Can you work these out from the model? Positions are in its coordinate system, mm. Give positions to 0.01 mm unless a question says otherwise; leave off trailing zeros. Write each loop counter-clockwise with the first axis right and the second up, starting at its lowest first coordinate (ties: lowest second). Pieces come first, ordered by that corner, then holes. Notation, with made-up numbers: (54.25, 4) -> (95.25, 4) arc R11 ccw to (95.25, 11) -> close; hole circle Ø9 at (49, 6). An arc over 180 degrees is marked (long way). One line per item, written item: value.
from build123d import *

# Parameters (mm, degrees)
SKETCH_W               = 190
SKETCH_H               = 132
PAD_DEPTH              = 10
SKETCH001_R            = 2.75
HOLE_DEPTH             = 10.001
LINEARPATTERN_COUNT    = 2
LINEARPATTERN_PITCH    = 60
LINEARPATTERN001_COUNT = 2
LINEARPATTERN001_PITCH = 122
HOLE001_D              = 6.6
HOLE001_CSINK_D        = 12
HOLE001_CSINK_ANGLE    = 90
LINEARPATTERN002_COUNT = 2
LINEARPATTERN002_PITCH = 40
LINEARPATTERN003_COUNT = 2
LINEARPATTERN003_PITCH = 170
LINEARPATTERN004_COUNT = 2
LINEARPATTERN004_PITCH = 130
HOLE002_D              = 6.6
HOLE002_CSINK_D        = 12
HOLE002_CSINK_ANGLE    = 90
LINEARPATTERN005_COUNT = 2
LINEARPATTERN005_PITCH = 40
LINEARPATTERN006_COUNT = 2
LINEARPATTERN006_PITCH = 130
LINEARPATTERN007_COUNT = 2
LINEARPATTERN007_PITCH = 170
HOLE003_D              = 6.6
HOLE003_CSINK_D        = 12
HOLE003_CSINK_ANGLE    = 90
LINEARPATTERN008_COUNT = 2
LINEARPATTERN008_PITCH = 40
LINEARPATTERN009_COUNT = 2
LINEARPATTERN009_PITCH = 130
LINEARPATTERN010_COUNT = 2
LINEARPATTERN010_PITCH = 170
SKETCH005_R            = 2.75
HOLE004_DEPTH          = 10.001
HOLE005_D              = 6.6
HOLE005_CSINK_D        = 12
HOLE005_CSINK_ANGLE    = 90
LINEARPATTERN011_COUNT = 2
LINEARPATTERN011_PITCH = 40
LINEARPATTERN012_COUNT = 2
LINEARPATTERN012_PITCH = 130
LINEARPATTERN013_COUNT = 2
LINEARPATTERN013_PITCH = 170
HOLE006_D              = 5.5
HOLE006_CSINK_D        = 10
HOLE006_CSINK_ANGLE    = 90
LINEARPATTERN014_COUNT = 2
LINEARPATTERN014_PITCH = 40
LINEARPATTERN015_COUNT = 2
LINEARPATTERN015_PITCH = 22
HOLE007_D              = 5.5
HOLE007_CSINK_D        = 10
HOLE007_CSINK_ANGLE    = 90


with BuildPart() as part:
    # Sketch → Pad (new body)
    with BuildSketch(Plane.XY):
        with Locations((95, 66)):
            Rectangle(SKETCH_W, SKETCH_H)
    extrude(amount=PAD_DEPTH)

    # Sketch001 (on Face6 of Pad) → Hole (cut, through all)
    with BuildSketch(Plane.XY.offset(10)):
        with Locations((65, 5)):
            Circle(SKETCH001_R)
    hole = extrude(amount=-HOLE_DEPTH, mode=Mode.SUBTRACT)

    # LinearPattern: Hole ×2
    with Locations(*[(i * LINEARPATTERN_PITCH, 0, 0) for i in range(1, LINEARPATTERN_COUNT)]):
        add(hole, mode=Mode.SUBTRACT)

    # LinearPattern001: Hole ×2
    with Locations(*[(0, i * LINEARPATTERN001_PITCH, 0) for i in range(1, LINEARPATTERN001_COUNT)]):
        add(hole, mode=Mode.SUBTRACT)

    # Hole001 (through all)
    with Locations(Plane.XY.offset(10)):
        with Locations((10, 18)):
            hole001 = CounterSinkHole(HOLE001_D / 2, HOLE001_CSINK_D / 2, counter_sink_angle=HOLE001_CSINK_ANGLE)

    # LinearPattern002: Hole001 ×2
    with Locations(*[(i * LINEARPATTERN002_PITCH, 0, 0) for i in range(1, LINEARPATTERN002_COUNT)]):
        add(hole001, mode=Mode.SUBTRACT)

    # LinearPattern003: Hole001 ×2
    with Locations(*[(i * LINEARPATTERN003_PITCH, 0, 0) for i in range(1, LINEARPATTERN003_COUNT)]):
        add(hole001, mode=Mode.SUBTRACT)

    # LinearPattern004: Hole001 ×2
    with Locations(*[(i * LINEARPATTERN004_PITCH, 0, 0) for i in range(1, LINEARPATTERN004_COUNT)]):
        add(hole001, mode=Mode.SUBTRACT)

    # Hole002 (through all)
    with Locations(Plane.XY.offset(10)):
        with Locations((10, 58)):
            hole002 = CounterSinkHole(HOLE002_D / 2, HOLE002_CSINK_D / 2, counter_sink_angle=HOLE002_CSINK_ANGLE)

    # LinearPattern005: Hole002 ×2
    with Locations(*[(i * LINEARPATTERN005_PITCH, 0, 0) for i in range(1, LINEARPATTERN005_COUNT)]):
        add(hole002, mode=Mode.SUBTRACT)

    # LinearPattern006: Hole002 ×2
    with Locations(*[(i * LINEARPATTERN006_PITCH, 0, 0) for i in range(1, LINEARPATTERN006_COUNT)]):
        add(hole002, mode=Mode.SUBTRACT)

    # LinearPattern007: Hole002 ×2
    with Locations(*[(i * LINEARPATTERN007_PITCH, 0, 0) for i in range(1, LINEARPATTERN007_COUNT)]):
        add(hole002, mode=Mode.SUBTRACT)

    # Hole003 (through all)
    with Locations(Plane.XY.offset(10)):
        with Locations((10, 114)):
            hole003 = CounterSinkHole(HOLE003_D / 2, HOLE003_CSINK_D / 2, counter_sink_angle=HOLE003_CSINK_ANGLE)

    # LinearPattern008: Hole003 ×2
    with Locations(*[(i * LINEARPATTERN008_PITCH, 0, 0) for i in range(1, LINEARPATTERN008_COUNT)]):
        add(hole003, mode=Mode.SUBTRACT)

    # LinearPattern009: Hole003 ×2
    with Locations(*[(i * LINEARPATTERN009_PITCH, 0, 0) for i in range(1, LINEARPATTERN009_COUNT)]):
        add(hole003, mode=Mode.SUBTRACT)

    # LinearPattern010: Hole003 ×2
    with Locations(*[(i * LINEARPATTERN010_PITCH, 0, 0) for i in range(1, LINEARPATTERN010_COUNT)]):
        add(hole003, mode=Mode.SUBTRACT)

    # Sketch005 (on Face5 of LinearPattern010) → Hole004 (cut, through all)
    with BuildSketch(Plane.XY.offset(10)):
        with Locations((125, 127)):
            Circle(SKETCH005_R)
    extrude(amount=-HOLE004_DEPTH, mode=Mode.SUBTRACT)

    # Hole005 (through all)
    with Locations(Plane.XY.offset(10)):
        with Locations((10, 74)):
            hole005 = CounterSinkHole(HOLE005_D / 2, HOLE005_CSINK_D / 2, counter_sink_angle=HOLE005_CSINK_ANGLE)

    # LinearPattern011: Hole005 ×2
    with Locations(*[(i * LINEARPATTERN011_PITCH, 0, 0) for i in range(1, LINEARPATTERN011_COUNT)]):
        add(hole005, mode=Mode.SUBTRACT)

    # LinearPattern012: Hole005 ×2
    with Locations(*[(i * LINEARPATTERN012_PITCH, 0, 0) for i in range(1, LINEARPATTERN012_COUNT)]):
        add(hole005, mode=Mode.SUBTRACT)

    # LinearPattern013: Hole005 ×2
    with Locations(*[(i * LINEARPATTERN013_PITCH, 0, 0) for i in range(1, LINEARPATTERN013_COUNT)]):
        add(hole005, mode=Mode.SUBTRACT)

    # Hole006 (through all)
    with Locations(Plane.XY.offset(10)):
        with Locations((75, 55)):
            hole006 = CounterSinkHole(HOLE006_D / 2, HOLE006_CSINK_D / 2, counter_sink_angle=HOLE006_CSINK_ANGLE)

    # LinearPattern014: Hole006 ×2
    with Locations(*[(i * LINEARPATTERN014_PITCH, 0, 0) for i in range(1, LINEARPATTERN014_COUNT)]):
        add(hole006, mode=Mode.SUBTRACT)

    # LinearPattern015: Hole006 ×2
    with Locations(*[(0, i * LINEARPATTERN015_PITCH, 0) for i in range(1, LINEARPATTERN015_COUNT)]):
        add(hole006, mode=Mode.SUBTRACT)

    # Hole007 (through all)
    with Locations(Plane.XY.offset(10)):
        with Locations((115, 77)):
            CounterSinkHole(HOLE007_D / 2, HOLE007_CSINK_D / 2, counter_sink_angle=HOLE007_CSINK_ANGLE)


solid = part.part
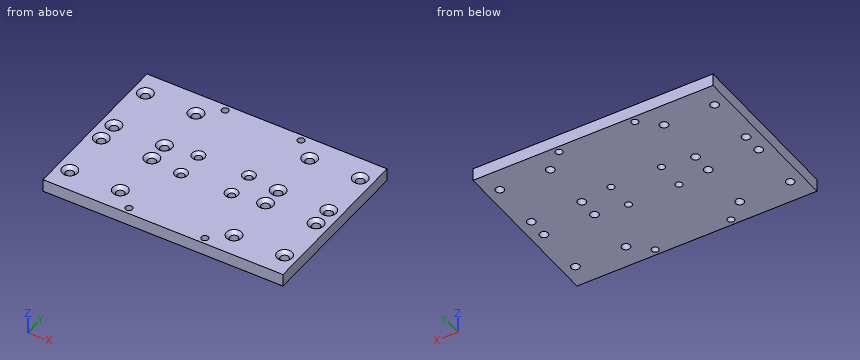
1) Will these pins go through, and if not, where does the flat tip stop? pin 1 (5 mm diameter, centred on x = 94.5, z = 5.5, fed in from -Y); pin 2 (10.5 mm diameter, centred on x = 50, y = 74, fed in from +Z); pin 3 (8.5 mm diameter, centred on x = 180, y = 74, fed in from +Z); pin 4 (7 mm diameter, centred on x = 115, y = 55, fed in from +Z).
Answer list:
pin 1: stops at y = 0
pin 2: stops at z = 9.25
pin 3: stops at z = 8.25
pin 4: stops at z = 8.5
2) If we section it at D-D (z = 4.75): State how many separate pieces and enclosed holes the cut face has, and give its area (3 significant figures).
Answer list:
separate pieces: 1
enclosed holes: 24
area: 24,300 mm^2
3) If we section it at B-B (y = 114): Write out the boundary of the cut face in (x, z).
Answer list:
outline: (0, 0) -> (6.7, 0) -> (6.7, 7.3) -> (4, 10) -> (0, 10) -> close; (13.3, 0) -> (46.7, 0) -> (46.7, 7.3) -> (44, 10) -> (16, 10) -> (13.3, 7.3) -> close; (53.3, 0) -> (136.7, 0) -> (136.7, 7.3) -> (134, 10) -> (56, 10) -> (53.3, 7.3) -> close; (143.3, 0) -> (176.7, 0) -> (176.7, 7.3) -> (174, 10) -> (146, 10) -> (143.3, 7.3) -> close; (183.3, 0) -> (190, 0) -> (190, 10) -> (186, 10) -> (183.3, 7.3) -> close
4) If we section it at A-A (x = 140): Write out the boundary of the cut face in (y, z), and give its area (3 significant figures).
Answer list:
outline: (0, 0) -> (14.7, 0) -> (14.7, 7.3) -> (12, 10) -> (0, 10) -> close; (21.3, 0) -> (54.7, 0) -> (54.7, 7.3) -> (52, 10) -> (24, 10) -> (21.3, 7.3) -> close; (61.3, 0) -> (70.7, 0) -> (70.7, 7.3) -> (68, 10) -> (64, 10) -> (61.3, 7.3) -> close; (77.3, 0) -> (110.7, 0) -> (110.7, 7.3) -> (108, 10) -> (80, 10) -> (77.3, 7.3) -> close; (117.3, 0) -> (132, 0) -> (132, 10) -> (120, 10) -> (117.3, 7.3) -> close
area: 1,030 mm^2
5) I need wall thicknesses on L1, parallel to X at y = 74, z = 4.75; L2, parallel to Y at x = 125, z = 4.25; L3, parallel to Y at x = 10, z = 5.25. Which ranges of each line are inside material? Lowest first, please.
Answer list:
L1: x = 0 to 6.7, 13.3 to 46.7, 53.3 to 136.7, 143.3 to 176.7, 183.3 to 190
L2: y = 0 to 2.25, 7.75 to 124.25, 129.75 to 132
L3: y = 0 to 14.7, 21.3 to 54.7, 61.3 to 70.7, 77.3 to 110.7, 117.3 to 132
6) If we section it at C-C (x = 115): Write out the boundary of the cut face in (y, z), and give its area (3 significant figures).
Answer list:
outline: (0, 0) -> (52.25, 0) -> (52.25, 7.75) -> (50, 10) -> (0, 10) -> close; (57.75, 0) -> (74.25, 0) -> (74.25, 7.75) -> (72, 10) -> (60, 10) -> (57.75, 7.75) -> close; (79.75, 0) -> (132, 0) -> (132, 10) -> (82, 10) -> (79.75, 7.75) -> close
area: 1,200 mm^2
